Autodesk Fusion 360 part; units mm, degrees
sketch "Sketch1" plane through (0, 0, 0) normal (0, 0, 1) x (1, 0, 0)
  arc A0 (29.5, -30.5) -> (35.5, -24.5) centre (29.5, -24.5) ccw
  arc A1 (35.5, 24.5) -> (29.5, 30.5) centre (29.5, 24.5) ccw
  circle A2 centre (29.5, 24.5) radius 1.5
  line L0 (-35.5, 24.5) -> (-35.5, -24.5)
  line L1 (29.5, -30.5) -> (-29.5, -30.5)
  line L2 (-29.5, 30.5) -> (29.5, 30.5)
  arc A3 (34, 25) -> (30, 29) centre (30, 25) ccw
  circle A4 centre (29.5, -24.5) radius 1.5
  arc A5 (30, -29) -> (34, -25) centre (30, -25) ccw
  line L3 (30, -29) -> (-30, -29)
  arc A6 (-34, -25) -> (-30, -29) centre (-30, -25) ccw
  line L4 (0, -27.5) -> (0.5, -27.5) construction
  arc A7 (-35.5, -24.5) -> (-29.5, -30.5) centre (-29.5, -24.5) ccw
  line L5 (-30, 29) -> (30, 29)
  arc A8 (-29.5, 30.5) -> (-35.5, 24.5) centre (-29.5, 24.5) ccw
  line L6 (0, 27.5) -> (0.5, 27.5) construction
  circle A9 centre (-29.5, 24.5) radius 1.5
  arc A10 (-30, 29) -> (-34, 25) centre (-30, 25) ccw
  line L7 (0, -27.5) -> (0.5, -27.5) construction
  line L8 (-34, -25) -> (-34, 25)
  circle A11 centre (-29.5, -24.5) radius 1.5
  line L9 (0, -27.5) -> (0.5, -27.5)
  arc A12 (-29.5, 30.5) -> (-35.5, 24.5) centre (-29.5, 24.5) ccw
  line L10 (34, 25) -> (34, -25)
  line L11 (35.5, 24.5) -> (35.5, -24.5)
  line L12 (-35.5, 0) -> (-30.5, 0) construction
  line L13 (-29, 8.5) -> (-29, 9.5) construction
  line L14 (-26.042, 8.5) -> (-31.958, 8.5)
  line L15 (-31.958, 7.5) -> (-26.042, 7.5)
  line L16 (-29, 8.5) -> (-29, 10) construction
  line L17 (-27.3417, 10.5) -> (-30.6583, 10.5)
  line L18 (-31.5981, 9.5) -> (-26.4019, 9.5)
  line L19 (-29, 7.5) -> (-29, 6) construction
  arc A13 (-30.6583, 10.5) -> (-31.5981, 9.5) centre (-29, 8) ccw
  arc A14 (-26.4019, 9.5) -> (-27.3417, 10.5) centre (-29, 8) ccw
  line L20 (-32, 8.5) -> (-31.9592, 8.4932) construction
  line L21 (-26.0408, 7.5068) -> (-26, 7.5) construction
  line L22 (-26.4019, 6.5) -> (-31.5981, 6.5)
  line L23 (-30.6583, 5.5) -> (-27.3417, 5.5)
  arc A15 (-31.958, 8.5) -> (-31.958, 7.5) centre (-29, 8) ccw
  arc A16 (-26.042, 7.5) -> (-26.042, 8.5) centre (-29, 8) ccw
  arc A17 (-31.5981, 6.5) -> (-30.6583, 5.5) centre (-29, 8) ccw
  arc A18 (-27.3417, 5.5) -> (-26.4019, 6.5) centre (-29, 8) ccw
  point P0 (-29, 8)
  point P1 (-29, 8)
  point P2 (-29, 10)
  point P3 (-29, 6)
  point P4 (-29, 6)
  dimension "d1" = 3
  dimension "d2" = 3
  dimension "d3" = 3
  dimension "d4" = 3
  dimension "d25" = 1.5
extrude "Extrude3" add sketch "Sketch1" along normal blind 2 contours A0 A1 L0 L1 L2 A7 A8 A12 L11
fillet "Fillet1" radius 1 8 edges at (-33.7426, 28.7426, 2) (-35.5, 0, 2) (-33.7426, -28.7426, 2) (0, -30.5, 2) (33.7426, -28.7426, 2) (35.5, 0, 2) (33.7426, 28.7426, 2) (0, 30.5, 2)
extrude "Extrude4" add sketch "Sketch1" along normal blind 1.5 contours A3 A5 L3 A6 L5 A10 L8 L10
extrude "Extrude2" [suppressed]
Geometry: final body of the model. Coordinates: model frame, mm. A direction names the side the tool comes from. Coordinates: 2 decimals unless noted, no trailing zeros. Order: outer loops, then holes, each group sorted by start corner. A loop starts at its lowest first (then second) coordinate and runs counter-clockwise, first axis right, second up.
(1) Access query for faces 4 (the face through (-29, 8.5, 1)), 5 (the face through (-33.789, 28.696, 0.493)), 6 (the face through (-32.797, -27.859, 1.746)). Directions: +Z, -Z, +X, -X, +Y, -Y. A direction counts if a zero-diameter tool reaches every point of the face in a straight line with its end or side. Return the directions, or none.
(2) Material intervals for probe 1 along Y at (x, z) = (-29.5, 0.4); probe 2 along Y at (x, z) = (29.5, 0.6); probe 3 along X at (y, z) = (24, 0.9), sorted ascending.
(3) Section query A-A (y = 1). Return the cut outline in (x, z).
(4) Draft query along Y for faces 1 (the face through (-33.696, -28.789, 0.493)), 2 (the face through (33.696, 28.789, 0.493)), 3 (the face through (-29, 6.5, 1)). Return one class per face: pulls with the +Y half, pulls with the -Y half, needs draft (parallel to the pull), parting line crosses it, or undercut.
(5) First-contact query: pin 1 (1.8 mm diameter, centred on x = 29.5, y = 24.5, fed in from +Z); pin 2 (4 mm diameter, centred on x = -29.5, y = 24.5, fed in from -Z). Flat tips, straight axial feed; report the tip coordinate or a pass-through.
(6) Section query B-B (x = 18.5). Return the cut outline in (y, z), plus the area to 3 significant figures.
Solution:
1. face 4: +Z, -Z
1. face 5: +Z, -Z, -X, +Y
1. face 6: +Z
2. probe 1: y = -30.5 to -26, -23 to 5.5, 6.5 to 7.5, 8.5 to 9.5, 10.5 to 23, 26 to 30.5
2. probe 2: y = -30.5 to -26, -23 to 23, 26 to 30.5
2. probe 3: x = -35.5 to -30.91, -28.09 to 28.09, 30.91 to 35.5
3. outline: (-35.5, 0) - (35.5, 0) - (35.5, 1) arc R1 ccw to (34.5, 2) - (34, 2) - (34, 1.5) - (-34, 1.5) - (-34, 2) - (-34.5, 2) arc R1 ccw to (-35.5, 1) - close
4. face 1: pulls with the -Y half
4. face 2: pulls with the +Y half
4. face 3: undercut
5. pin 1: passes through
5. pin 2: stops at z = 0
6. outline: (-30.5, 0) - (30.5, 0) - (30.5, 1) arc R1 ccw to (29.5, 2) - (29, 2) - (29, 1.5) - (-29, 1.5) - (-29, 2) - (-29.5, 2) arc R1 ccw to (-30.5, 1) - close
6. area: 92.6 mm2
